```python
from build123d import *

# Parameters (mm, degrees)
EXTRUDE_THIN1_DEPTH = 25.4
SKETCH3_R           = 3.021976596
EXTRUDE2_DEPTH      = 82.338554141
SKETCH4_R           = 3.556
EXTRUDE3_DEPTH      = 81.534
FILLET1_R           = 6.35


with BuildPart() as part:
    # Sketch1 → Extrude-Thin1 (new body)
    with BuildSketch(Plane.XY):
        with BuildLine():
            Line((0, 22.225), (0, 3.175))
            ThreePointArc((0, 3.175), (0.92993597, 0.92993597), (3.175, 0))
            Line((3.175, 0), (68.290741431, 0))
            ThreePointArc((68.290741431, 0), (70.535805461, 0.92993597), (71.465741431, 3.175))
            Line((71.465741431, 3.175), (71.465741431, 22.225))
            Line((71.465741431, 22.225), (74.005741431, 22.225))
            Line((74.005741431, 22.225), (74.005741431, 3.175))
            ThreePointArc((74.005741431, 3.175), (72.331856686, -0.866115254), (68.290741431, -2.54))
            Line((68.290741431, -2.54), (3.175, -2.54))
            ThreePointArc((3.175, -2.54), (-0.866115254, -0.866115254), (-2.54, 3.175))
            Line((-2.54, 3.175), (-2.54, 22.225))
            Line((-2.54, 22.225), (0, 22.225))
        make_face()
    extrude(amount=EXTRUDE_THIN1_DEPTH)

    # Sketch3 → Extrude2 (cut, through all)
    with BuildSketch(Plane(origin=(0, 0, 0), x_dir=(1, 0, 0), z_dir=(0, 1, 0))):
        with Locations(Location((18.493278585, -12.7, 0), (0, 0, 270))):
            Circle(SKETCH3_R)
        with Locations(Location((52.972462846, -12.7, 0), (0, 0, 90))):
            Circle(SKETCH3_R)
    extrude(amount=-EXTRUDE2_DEPTH, mode=Mode.SUBTRACT)

    # Sketch4 → Extrude3 (cut, symmetric)
    with BuildSketch(Plane(origin=(0, 0, 0), x_dir=(0, 0, -1), z_dir=(1, 0, 0))):
        with Locations(Location((-12.7, 13.821871469, 0), (0, 0, 90))):
            Circle(SKETCH4_R)
    extrude(amount=EXTRUDE3_DEPTH, both=True, mode=Mode.SUBTRACT)

    # Fillet1
    fillet1_edges = [part.edges().sort_by_distance(p)[0] for p in [
        (-1.27, 22.225, 0),
        (72.735741431, 22.225, 0),
        (-1.27, 22.225, 25.4),
        (72.735741431, 22.225, 25.4),
    ]]
    fillet(fillet1_edges, radius=FILLET1_R)


solid = part.part
```
CAD build for the part. Positions are in the model's coordinates, mm. A direction names the side the tool comes from. Coordinates: 2 decimals unless noted, no trailing zeros. Loops run counter-clockwise (first coordinate to the right, second up) from the corner with the lowest first, then second, coordinate; pieces in that order, holes last. Notation, with made-up numbers: (5.25, 82) - (28.25, 82) arc R20 cw to (28.25, 96) - close; hole circle Ø1 at (-7.75, 21). An arc over 180 degrees is marked (long way). Use CSV: the item, a comma, the result in double quotes. Start each with the question number.
Q1. 3-axis set-ups, long thin cutter, end or side, ignore diameter. For faces 1 (the flat face through (73, 22.225, 13)), 2 (the cylindrical face through (70.511, 0.905, 12.522)): which of +Z, -Z, +X, -X, +Y, -Y reach the whole face in a straight line?
Q2. Cut at D-D, the plane x = 11. List the corners of the cut face in (y, z).
Q3. Cut at A-A, the plane z = 12.7. List the corners of the cut face in (x, y) (3 decimals).
Q4. Two-plate mould, pull along X, no slides. Class faces 3 (the flat face through (-2.54, 10, 15)), 4 (the cylindrical face through (0.91, 0.95, 12.52)), 5 (the cylindrical face through (-1.252, 20.414, 1.91)): +X half, -X half, draft (parallel to the pull), parting line (faces both ways), or undercut.
Q5. Drop flat-ended pins along their axis: P1, Ø1.5, axis at y = 1.5, z = 23, coming from the +X side; P2, Ø11.5, axis at y = 13.82, z = 12.7, coming from the -X side; P3, Ø3, axis at y = 0, z = 12.5, coming from the +X side; P4, Ø9.5, axis at x = 52.97, z = 12.7, coming from the +Y side. Give the stop position or say it passes through.
Q6. Cut at C-C, the plane z = 23. List the corners of the cut face in (x, y) (3 decimals), then the cut area to 3 significant figures.
Q7. Probe probe 1 along X at (y, z) = (7.5, 5); probe 2 along Y at (x, z) = (17.5, 19.5); probe 3 along X at (y, z) = (-1.5, 12.7). List the from-to ranges inside material, lowest first. Write a range as from..to.
Q8. Cut at B-B, the plane y = 20.5. List the corners of the cut face in (x, z), then the cut area to 3 significant figures.
Here are the results:
1,face 1,"+Z, -Z, +X, -X, +Y"
1,face 2,"+Z, -Z, +Y"
2,outline,"(-2.54, 0) - (0, 0) - (0, 25.4) - (-2.54, 25.4) - close"
3,outline,"(-2.54, 3.175) arc R5.715 ccw to (3.175, -2.54) - (15.471, -2.54) - (15.471, 0) - (3.175, 0) arc R3.175 cw to (0, 3.175) - (0, 10.266) - (-2.54, 10.266) - close; (-2.54, 17.378) - (0, 17.378) - (0, 22.225) - (-2.54, 22.225) - close; (21.515, -2.54) - (49.95, -2.54) - (49.95, 0) - (21.515, 0) - close; (55.994, -2.54) - (68.291, -2.54) arc R5.715 ccw to (74.006, 3.175) - (74.006, 10.266) - (71.466, 10.266) - (71.466, 3.175) arc R3.175 cw to (68.291, 0) - (55.994, 0) - close; (71.466, 17.378) - (74.006, 17.378) - (74.006, 22.225) - (71.466, 22.225) - close"
4,face 3,"-X half"
4,face 4,"undercut"
4,face 5,"draft"
5,P1,"x = 73.93"
5,P2,"x = -2.54"
5,P3,"x = 73.75"
5,P4,"y = 0"
6,outline,"(-2.54, 3.175) arc R5.715 ccw to (3.175, -2.54) - (68.291, -2.54) arc R5.715 ccw to (74.006, 3.175) - (74.006, 20.847) - (71.466, 20.847) - (71.466, 3.175) arc R3.175 cw to (68.291, 0) - (3.175, 0) arc R3.175 cw to (0, 3.175) - (0, 20.847) - (-2.54, 20.847) - close"
6,area,"291 mm2"
7,probe 1,"-2.54..0, 71.47..74.01"
7,probe 2,"-2.54..0"
7,probe 3,"-0.11..15.47, 21.52..49.95, 55.99..71.58"
8,outline,"(-2.54, 2) - (0, 2) - (0, 23.4) - (-2.54, 23.4) - close; (71.47, 2) - (74.01, 2) - (74.01, 23.4) - (71.47, 23.4) - close"
8,area,"109 mm2"
